Autodesk Inventor part; units mm, degrees
ref_plane "YZ Plane" through (0, 0, 0) normal (1, 0, 0) x (0, 1, 0)
ref_plane "XZ Plane" through (0, 0, 0) normal (0, 1, 0) x (-1, 0, 0)
ref_plane "XY Plane" through (0, 0, 0) normal (0, 0, 1) x (1, 0, 0)
sketch "Sketch2" plane through (0, 0, 0) normal (1, 0, 0) x (0, 1, 0)
  line L0 (0, 0) -> (3, 0) construction
  line L1 (3, -3) -> (3, -50)
  line L2 (3, -50) -> (0, -50)
  line L3 (0, -50) -> (0, -120)
  line L4 (0, -120) -> (3, -120)
  line L5 (53, 0) -> (53, -3)
  line L6 (33, -3) -> (33, 0)
  line L7 (0, 0) -> (0, -43) construction
  line L8 (0, -43) -> (15, -43) construction
  line L9 (15, -43) -> (35, -43) construction
  line L10 (15, -43) -> (15, -63)
  line L11 (15, -63) -> (35, -63)
  line L12 (35, -63) -> (35, -43)
  line L13 (35, -43) -> (15, -43)
  line L14 (83, -164) -> (83, -117)
  line L15 (3, -167) -> (3, -120)
  line L16 (3, -167) -> (33, -167)
  line L17 (33, -167) -> (33, -170)
  line L18 (33, -170) -> (53, -170)
  line L19 (53, -170) -> (53, -167)
  line L20 (53, -167) -> (83, -167)
  line L21 (83, -167) -> (83, -164)
  line L22 (53, -3) -> (83, -3)
  line L23 (53, 0) -> (33, 0)
  line L24 (33, -3) -> (3, -3)
  line L25 (83, -3) -> (83, -117)
  dimension "d0" = 3
  dimension "d1" = 3
  dimension "d2" = 47
  dimension "d3" = 70
  dimension "d11" = 3
  dimension "d12" = 20
  dimension "d15" = 43
  dimension "d16" = 15
  dimension "d17" = 20
  dimension "d18" = 20
  dimension "d19" = 47
  dimension "d20" = 30
  dimension "d21" = 3
  dimension "d22" = 20
extrude "Extrusion1" add sketch "Sketch2" along normal blind 3
properties part number "Kiri"
Model file for the job. Use its own axes, mm. A direction names the side the tool comes from. Coordinates: 2 decimals unless noted, no trailing zeros. Loops run counter-clockwise (first coordinate to the right, second up) from the corner with the lowest first, then second, coordinate; pieces in that order, holes last. Notation, with made-up numbers: M 15.5,25.25 L 36.5,25.25 A29 cw 36.5,52.25 Z; hole C -17,64 d11. An arc over 180 degrees is marked long. Use CSV: the item, a comma, the result in double quotes. Start each with the question number.
1. Band-saw the part on C-C, the plane y = 31. List the corners of the cut face in (x, z).
2. Flat gauge pins, fed straight in: pin 1 (0.9 mm diameter, centred on x = 2, z = -168.5, fed in from -Y); pin 2 (0.9 mm diameter, centred on x = 1, z = -169, fed in from +Y); pin 3 (1.5 mm diameter, centred on x = 1, y = 1, fed in from +Z). Where does each tip first touch, or does it go through?
3. Band-saw the part on B-B, the plane x = 1.55. List the corners of the cut face in (y, z).
4. Two-plate mould, pull along Y, no slides. Class faces 5 (the flat face through (1, 25, -63)), 6 (the flat face through (1, 2, -50)), 7 (the flat face through (1, 83, -84)), 8 (the flat face through (1, 3, -26)): pulls with the +Y half, pulls with the -Y half, needs draft (parallel to the pull), parting line crosses it, or undercut.
5. Tool access for faces 1 (the flat face through (1, 3, -144)), 2 (the flat face through (1, 53, -169)), 3 (the flat face through (1, 25, -43)), 4 (the flat face through (1, 18, -3)): list every direction of +Z, -Z, +X, -X, +Y, -Y with a clear straight run to the whole face (end or side of a thin tool).
6. Probe probe 1 along Y at (x, z) = (0.6, -62); probe 2 along Y at (x, z) = (2, -48.5); probe 3 along Z at (x, y) = (2.7, 31). List the from-to ranges inside material, lowest first. Write a range as [from, to].
7. Band-saw the part on A-A, the plane z = -46. List the corners of the cut face in (x, y).
8. Band-saw the part on D-D, the plane y = 59. List the corners of the cut face in (x, z), then the cut area to 3 significant figures.
Entries:
1,outline,"M 0,-167 L 3,-167 L 3,-63 L 0,-63 Z; M 0,-43 L 3,-43 L 3,-3 L 0,-3 Z"
2,pin 1,"stops at y = 33"
2,pin 2,"stops at y = 53"
2,pin 3,"stops at z = -50"
3,outline,"M 0,-120 L 3,-120 L 3,-167 L 33,-167 L 33,-170 L 53,-170 L 53,-167 L 83,-167 L 83,-3 L 53,-3 L 53,0 L 33,0 L 33,-3 L 3,-3 L 3,-50 L 0,-50 Z; hole M 15,-63 L 35,-63 L 35,-43 L 15,-43 Z"
4,face 5,"undercut"
4,face 6,"needs draft"
4,face 7,"pulls with the +Y half"
4,face 8,"pulls with the -Y half"
5,face 1,"-Z, +X, -X, -Y"
5,face 2,"-Z, +X, -X, +Y"
5,face 3,"+X, -X"
5,face 4,"+Z, +X, -X, -Y"
6,probe 1,"y = [0, 15], [35, 83]"
6,probe 2,"y = [3, 15], [35, 83]"
6,probe 3,"z = [-167, -63], [-43, -3]"
7,outline,"M 0,3 L 3,3 L 3,15 L 0,15 Z; M 0,35 L 3,35 L 3,83 L 0,83 Z"
8,outline,"M 0,-167 L 3,-167 L 3,-3 L 0,-3 Z"
8,area,"492 mm2"
